from build123d import *

# Parameters (mm, degrees)
EXTRUDE_DEPTH = 4.7


with BuildPart() as revolve_body:
    # Sketch001 → Revolve (revolve)
    with BuildSketch(Plane.XZ):
        Polygon((3, 0), (2.5, 0.288675), (2.5, 0.561325), (3, 0.85), (2.5, 1.138675), (2.5, 1.561325), (3, 1.85), (2.5, 2.138675), (2.5, 2.561325), (3, 2.85), (2.5, 3.138675), (2.5, 3.561325), (3, 3.85), (2.5, 4.138675), (2.5, 4.411325), (3, 4.7), (4.9, 4.7), (6, 4.064915), (6, 0.635085), (4.9, 0), align=None)
    revolve(axis=Axis((0, 0, 0), (0, 0, 1)))


with BuildPart() as common:
    # Sketch → Extrude (new body)
    with BuildSketch(Plane.XY):
        Polygon((0, 5.773503), (-5, 2.886751), (-5, -2.886751), (0, -5.773503), (5, -2.886751), (5, 2.886751), align=None)
    extrude(amount=EXTRUDE_DEPTH)

    # Common: intersect Revolve body
    add(revolve_body.part, mode=Mode.INTERSECT)


solid = common.part
Check sheet for the modelled part. Datum: model origin and axes. Units: mm. Round coordinates to 2 decimals unless told otherwise and drop trailing zeros. Write each loop counter-clockwise with the first axis right and the second up, starting at its lowest first coordinate (ties: lowest second). Pieces come first, ordered by that corner, then holes. Notation, with made-up numbers: (-33, -2.75) - (-15, -2.75) arc R11 cw to (-15, 7.25) - close; hole circle Ø9 at (74, 45.25). An arc over 180 degrees is marked (long way). Return JSON: item names as keys, results as strings.
Q1. Scan lines: L1, parallel to Y at x = 1.75, z = 1.6; L2, parallel to X at y = 1, z = 2.25; L3, parallel to Y at x = 1.5, z = 0.75. Record each from-to range of solid material in increasing order. Write a range as from..to.
Returned:
{"L1": "y = -4.76..-1.88, 1.88..4.76", "L2": "x = -5..-2.29, 2.29..5", "L3": "y = -4.91..-2.4, 2.4..4.91"}
Q2. Cross-section at A-A (z = 1.3). Record the boundary of the cut face in (x, y), then the cut area to 3 significant figures.
Returned:
{"outline": "(-5, -2.89) - (0, -5.77) - (5, -2.89) - (5, 2.89) - (0, 5.77) - (-5, 2.89) - close; hole circle Ø5 at (0, 0)", "area": "67.0 mm²"}
Q3. Depth check by flat-ended pin: P1, Ø1, axis at y = 3.5, z = 1.5, coming from the -X side. Enter the tip coordinate at first touch or a pass-through.
Returned:
{"P1": "stops at x = -4.8"}
